from build123d import *

# Parameters (mm, degrees)
SCHIZZO1_W                   = 150
SCHIZZO1_H                   = 55
ESTRUSIONE_ESTRUSIONE1_DEPTH = 1.7
SCHIZZO2_W                   = 98
SCHIZZO2_H                   = 60
ESTRUSIONE_ESTRUSIONE2_DEPTH = 4
SCHIZZO3_W                   = 98
SCHIZZO3_H                   = 40
ESTRUSIONE_ESTRUSIONE3_DEPTH = 10


with BuildPart() as part:
    # Schizzo1 → Estrusione-Estrusione1 (new body)
    with BuildSketch(Plane.XY):
        Rectangle(SCHIZZO1_W, SCHIZZO1_H)
    extrude(amount=ESTRUSIONE_ESTRUSIONE1_DEPTH)

    # Schizzo2 → Estrusione-Estrusione2 (add)
    with BuildSketch(Plane.XY.offset(1.7)):
        with Locations((-12, -5.5)):
            Rectangle(SCHIZZO2_W, SCHIZZO2_H)
    extrude(amount=ESTRUSIONE_ESTRUSIONE2_DEPTH)

    # Schizzo3 → Estrusione-Estrusione3 (add)
    with BuildSketch(Plane.XY.offset(5.7)):
        with Locations((-12, -5.5)):
            Rectangle(SCHIZZO3_W, SCHIZZO3_H)
    extrude(amount=ESTRUSIONE_ESTRUSIONE3_DEPTH)


solid = part.part
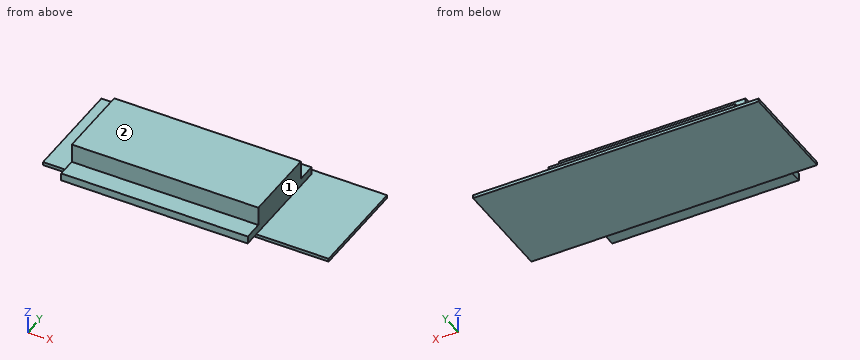
Verification items for the finished model (mm, model axes). Face numbers are marked on the shaded views. A direction names the side the tool comes from. Coordinates: 2 decimals unless noted, no trailing zeros. Loops run counter-clockwise (first coordinate to the right, second up) from the corner with the lowest first, then second, coordinate; pieces in that order, holes last. Notation, with made-up numbers: (-35, 77) -> (-15, 77) arc R38 ccw to (-15, 115) -> close; hole circle Ø9 at (38.25, 16.25). An arc over 180 degrees is marked (long way). Answer as a JSON object with one key per item and string values. Group by question number.
Item 1: Depth check by flat-ended pin: pin 1 (2 mm diameter, centred on x = 28.5, z = 7.5, fed in from -Y); pin 2 (5 mm diameter, centred on x = -15, z = 5.5, fed in from +Y); pin 3 (5 mm diameter, centred on y = -11, z = 12, fed in from +X). Enter the tip coordinate at first touch or a pass-through.
Item 2: Sectioned sample at A-A on x = -55. Record the boundary of the cut face in (y, z).
Item 3: Scan lines: probe 1 along Z at (x, y) = (-43, 25); probe 2 along X at (y, z) = (-6, 2.25); probe 3 along Y at (x, z) = (-38.5, 2.75). Record each from-to range of solid material in increasing order.
Item 4: Tool access check on the marked faces 1 and 2. Record the directions out of +Z, -Z, +X, -X, +Y, -Y that give a thin tool (end or side, any length) a straight path to the whole face; none if there is none.
Item 5: Sectioned sample at D-D on x = 65. Record the boundary of the cut face in (y, z).
Item 6: Sectioned sample at C-C on z = 10.5. Record the boundary of the cut face in (x, y), plus the area to 3 significant figures.
Item 7: Sectioned sample at B-B on y = 7. Record the boundary of the cut face in (x, z).
Evaluation:
{
 "1": {"pin 1": "stops at y = -25.5", "pin 2": "stops at y = 24.5", "pin 3": "stops at x = 37"},
 "2": {"outline": "(-35.5, 1.7) -> (-27.5, 1.7) -> (-27.5, 0) -> (27.5, 0) -> (27.5, 1.7) -> (24.5, 1.7) -> (24.5, 5.7) -> (14.5, 5.7) -> (14.5, 15.7) -> (-25.5, 15.7) -> (-25.5, 5.7) -> (-35.5, 5.7) -> close"},
 "3": {"probe 1": "z = 0 to 1.7", "probe 2": "x = -61 to 37", "probe 3": "y = -35.5 to 24.5"},
 "4": {"face 1": "+Z, +X, +Y, -Y", "face 2": "+Z, +X, -X, +Y, -Y"},
 "5": {"outline": "(-27.5, 0) -> (27.5, 0) -> (27.5, 1.7) -> (-27.5, 1.7) -> close"},
 "6": {"outline": "(-61, -25.5) -> (37, -25.5) -> (37, 14.5) -> (-61, 14.5) -> close", "area": "3,920 mm²"},
 "7": {"outline": "(-75, 0) -> (75, 0) -> (75, 1.7) -> (37, 1.7) -> (37, 15.7) -> (-61, 15.7) -> (-61, 1.7) -> (-75, 1.7) -> close"}
}
